Work out the finished part from the listing and answer in its coordinate system (mm). Face numbers are marked on the shaded views. A direction names the side the tool comes from. Round coordinates to 2 decimals unless told otherwise and drop trailing zeros. Write each loop counter-clockwise with the first axis right and the second up, starting at its lowest first coordinate (ties: lowest second). Pieces come first, ordered by that corner, then holes.
from build123d import *

# Parameters (mm, degrees)
BOSS_EXTRUDE10_DEPTH = 3
SKETCH12_W           = 3
SKETCH12_H           = 12
BOSS_EXTRUDE11_DEPTH = 48
BOSS_EXTRUDE12_REACH = 39.563
SKETCH13_W           = 3
SKETCH13_H           = 12
CUT_EXTRUDE1_DEPTH   = 3
BOSS_EXTRUDE13_DEPTH = 6
CUT_EXTRUDE2_REACH   = 36.536
SKETCH16_R           = 2.2733


with BuildPart() as part:
    # Sketch10 → Boss-Extrude10 (new body)
    with BuildSketch(Plane(origin=(25.395802875, 0, 0), x_dir=(0, 0, -1), z_dir=(1, 0, 0))):
        Polygon((12.569444444, -3.3), (15.569444444, -3.3), (15.569444444, 8.7), (12.569444444, 8.7), (-7.430555556, 8.7), (-10.430555556, 8.7), (-10.430555556, -3.3), (-7.430555556, -3.3), align=None)
    extrude(amount=BOSS_EXTRUDE10_DEPTH)

    # Sketch12 → Boss-Extrude11 (add)
    with BuildSketch(Plane.ZY.offset(-25.395802875)):
        with Locations((-14.069444444, 2.7)):
            Rectangle(SKETCH12_W, SKETCH12_H)
        with Locations((8.930555556, 2.7)):
            Rectangle(SKETCH12_W, SKETCH12_H)
    extrude(amount=BOSS_EXTRUDE11_DEPTH)

    # Sketch13 → Boss-Extrude12 (add, up to next)
    with BuildSketch(Plane.XY.offset(-12.569444444), mode=Mode.PRIVATE) as boss_extrude12_sk1:
        with Locations((-21.104197125, 2.7)):
            Rectangle(SKETCH13_W, SKETCH13_H)
    boss_extrude12_tool1 = extrude(boss_extrude12_sk1.sketch, amount=BOSS_EXTRUDE12_REACH, mode=Mode.PRIVATE) - part.part
    add(boss_extrude12_tool1.solids().sort_by_distance((-21.104197, 2.7, -12.569444))[0])

    # Sketch14 → Cut-Extrude1 (cut)
    with BuildSketch(Plane.XY.offset(10.430555556)):
        Polygon((2.895802875, 8.7), (14.895802875, 8.7), (14.895802875, -3.3), (-9.104197125, -3.3), (-9.104197125, 8.7), align=None)
    extrude(amount=-CUT_EXTRUDE1_DEPTH, mode=Mode.SUBTRACT)

    # Sketch15 → Boss-Extrude13 (add)
    with BuildSketch(Plane.XZ.offset(3.3)):
        Polygon((-22.604197125, 10.430555556), (-22.604197125, -15.569444444), (28.395802875, -15.569444444), (28.395802875, 10.430555556), (14.895802875, 10.430555556), (14.895802875, 7.430555556), (14.895802875, 1.430555556), (-9.104197125, 1.430555556), (-9.104197125, 7.430555556), (-9.104197125, 10.430555556), align=None)
    extrude(amount=BOSS_EXTRUDE13_DEPTH)

    # Sketch16 → Cut-Extrude2 (cut, up to next)
    with BuildSketch(Plane(origin=(0, -3.3, 0), x_dir=(1, 0, 0), z_dir=(0, 1, 0)), mode=Mode.PRIVATE) as cut_extrude2_sk1:
        with Locations(Location((-9.104197125, 5.569444444, 0), (0, 0, 270))):
            Circle(SKETCH16_R)
    cut_extrude2_tool1 = extrude(cut_extrude2_sk1.sketch, amount=-CUT_EXTRUDE2_REACH, mode=Mode.PRIVATE) & part.part
    # Sketch16 → Cut-Extrude2 (cut, up to next)
    with BuildSketch(Plane(origin=(0, -3.3, 0), x_dir=(1, 0, 0), z_dir=(0, 1, 0)), mode=Mode.PRIVATE) as cut_extrude2_sk2:
        with Locations(Location((14.895802875, 5.569444444, 0), (0, 0, 270))):
            Circle(SKETCH16_R)
    cut_extrude2_tool2 = extrude(cut_extrude2_sk2.sketch, amount=-CUT_EXTRUDE2_REACH, mode=Mode.PRIVATE) & part.part
    add(cut_extrude2_tool1.solids().sort_by_distance((-9.104197, -3.3, -5.569444))[0], mode=Mode.SUBTRACT)
    add(cut_extrude2_tool2.solids().sort_by_distance((14.895803, -3.3, -5.569444))[0], mode=Mode.SUBTRACT)


solid = part.part
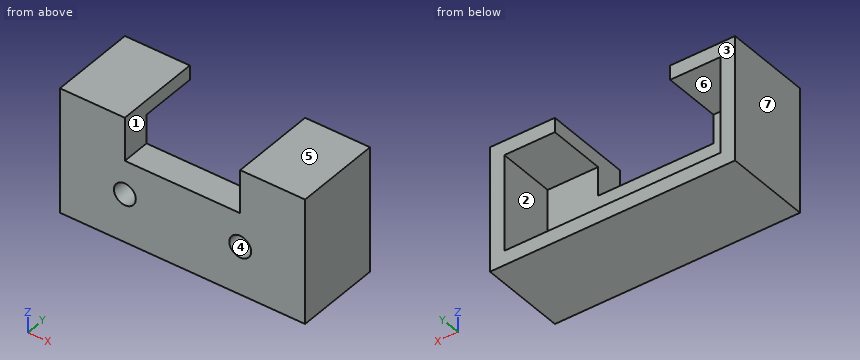
Q1. Find section D-D (z = 0.5). Determine the outline of the cut face in (x, y).
Q2. Find section B-B (y = -5). Determine the outline of the cut face in (x, z), plus the area to 3 significant figures.
Q3. The mould has two halves that part along X. Classify the marked faces 4, 5, 6 and 7: +X half, -X half, draft (parallel to the pull), parting line (faces both ways), or undercut.
Q4. Find section C-C (x = 15.5). Determine the outline of the cut face in (y, z).
Q5. Given pin 1 (3.5 mm diameter, centred on x = 10.5, y = 1.5, fed in from +Z); pin 2 (6.5 mm diameter, centred on x = 2, y = -5.5, fed in from +Z); pin 3 (2.5 mm diameter, centred on x = -9.1, z = -5.57, fed in from +Y), each flat-ended and moving along its own axis, determine where each tip first touches the part or whether it passes through.
Q6. Find the intervals of material crossed by L1, parallel to Z at x = 16, y = 2.75; L2, parallel to X at y = 2, z = 7.75; L3, parallel to X at y = -0.5, z = 1.75, in increasing order.
Q7. A tool of negligible diameter and unlimited length cuts with its end or side. For the marked faces 1, 2 and 3, from which of +Z, -Z, +X, -X, +Y, -Y can it reach the whole face along a straight path? Write none if from no direction.
Q8. Find section A-A (z = 5.5). Determine the outline of the cut face in (x, y), plus the area to 3 significant figures.
Report:
1. outline: (-22.6, -9.3) - (28.4, -9.3) - (28.4, 8.7) - (25.4, 8.7) - (25.4, -3.3) - (-19.6, -3.3) - (-19.6, 8.7) - (-22.6, 8.7) - close
2. outline: (-22.6, -15.57) - (28.4, -15.57) - (28.4, 10.43) - (14.9, 10.43) - (14.9, 1.43) - (-9.1, 1.43) - (-9.1, 10.43) - (-22.6, 10.43) - close; hole circle Ø4.55 at (-9.1, -5.57); hole circle Ø4.55 at (14.9, -5.57)
2. area: 1,080 mm2
3. face 4: undercut
3. face 5: draft
3. face 6: undercut
3. face 7: -X half
4. outline: (-9.3, -15.57) - (8.7, -15.57) - (8.7, -12.57) - (-3.3, -12.57) - (-3.3, -7.76) - (-9.3, -7.76) - close; (-9.3, -3.38) - (-3.3, -3.38) - (-3.3, 7.43) - (8.7, 7.43) - (8.7, 10.43) - (-9.3, 10.43) - close
5. pin 1: stops at z = -12.57
5. pin 2: stops at z = 1.43
5. pin 3: passes through
6. L1: z = -15.57 to -12.57, 7.43 to 10.43
6. L2: x = -22.6 to -9.1, 14.9 to 28.4
6. L3: x = -22.6 to -19.6, 25.4 to 28.4
7. face 1: +Z, +Y, -Y
7. face 2: +Y
7. face 3: +Z, -Z, +X, -X, +Y
8. outline: (-22.6, -9.3) - (-9.1, -9.3) - (-9.1, -3.3) - (-19.6, -3.3) - (-19.6, 8.7) - (-22.6, 8.7) - close; (14.9, -9.3) - (28.4, -9.3) - (28.4, 8.7) - (25.4, 8.7) - (25.4, -3.3) - (14.9, -3.3) - close
8. area: 234 mm2
